```python
from build123d import *

# Parameters (mm, degrees)
F0_W        = 88.9
F0_H        = 165.1
F1_DEPTH    = 6.35
F2_DEPTH    = 25.4
F3_DEPTH    = 50.8
F4_C1_SIZE2 = 7.3323484187
F4_C1_SIZE  = 12.7
F4_C2_SIZE2 = 7.3323484187
F4_C2_SIZE  = 12.7
F4_C3_SIZE2 = 12.7
F4_C3_SIZE  = 7.3323484187
F4_C4_SIZE2 = 12.7
F4_C4_SIZE  = 7.3323484187
F5_R        = 6.34999
F6_C1_SIZE2 = 7.3323484187
F6_C1_SIZE  = 12.7
F6_C2_SIZE2 = 7.3323484187
F6_C2_SIZE  = 12.7
F6_C3_SIZE2 = 12.7
F6_C3_SIZE  = 7.3323484187
F6_C4_SIZE2 = 12.7
F6_C4_SIZE  = 7.3323484187


# Not quite as in the source:
# - a fillet or chamfer is up to 0.001 mm smaller than in the source, because OpenCascade refuses the exact size


with BuildPart() as f1:
    # F0 (on Top) → F1 (new body)
    with BuildSketch(Plane.XY):
        Rectangle(F0_W, F0_H)
        Polygon((0, 76.2), (38.1, 76.2), (38.1, -38.1), (38.1, -76.2), (0, -76.2), (-38.1, -76.2), (-38.1, 38.1), (-38.1, 76.2), align=None, mode=Mode.SUBTRACT)
        with BuildLine():
            Line((0, 50.8), (0, 76.2))
            Line((0, 76.2), (-38.1, 76.2))
            Line((-38.1, 76.2), (-38.1, 38.1))
            Line((-38.1, 38.1), (-12.7, 38.1))
            ThreePointArc((-12.7, 38.1), (-3.7197438789, 41.8197438789), (0, 50.8))
        make_face()
        with BuildLine():
            Line((38.1, -38.1), (38.1, 76.2))
            Line((38.1, 76.2), (0, 76.2))
            Line((0, 76.2), (0, 50.8))
            ThreePointArc((0, 50.8), (-3.7197438789, 41.8197438789), (-12.7, 38.1))
            Line((-12.7, 38.1), (-38.1, 38.1))
            Line((-38.1, 38.1), (-38.1, -76.2))
            Line((-38.1, -76.2), (0, -76.2))
            Line((0, -76.2), (0, -50.8))
            ThreePointArc((0, -50.8), (3.7197438789, -41.8197438789), (12.7, -38.1))
            Line((12.7, -38.1), (38.1, -38.1))
        make_face()
        with BuildLine():
            Line((38.1, -76.2), (38.1, -38.1))
            Line((38.1, -38.1), (12.7, -38.1))
            ThreePointArc((12.7, -38.1), (3.7197438789, -41.8197438789), (0, -50.8))
            Line((0, -50.8), (0, -76.2))
            Line((0, -76.2), (38.1, -76.2))
        make_face()
    extrude(amount=F1_DEPTH)

    # F0 (on Top) → F2 (join)
    with BuildSketch(Plane.XY):
        with BuildLine():
            Line((38.1, -38.1), (38.1, 76.2))
            Line((38.1, 76.2), (0, 76.2))
            Line((0, 76.2), (0, 50.8))
            ThreePointArc((0, 50.8), (-3.7197438789, 41.8197438789), (-12.7, 38.1))
            Line((-12.7, 38.1), (-38.1, 38.1))
            Line((-38.1, 38.1), (-38.1, -76.2))
            Line((-38.1, -76.2), (0, -76.2))
            Line((0, -76.2), (0, -50.8))
            ThreePointArc((0, -50.8), (3.7197438789, -41.8197438789), (12.7, -38.1))
            Line((12.7, -38.1), (38.1, -38.1))
        make_face()
        with BuildLine():
            Line((0, 50.8), (0, 76.2))
            Line((0, 76.2), (-38.1, 76.2))
            Line((-38.1, 76.2), (-38.1, 38.1))
            Line((-38.1, 38.1), (-12.7, 38.1))
            ThreePointArc((-12.7, 38.1), (-3.7197438789, 41.8197438789), (0, 50.8))
        make_face()
        with BuildLine():
            Line((38.1, -76.2), (38.1, -38.1))
            Line((38.1, -38.1), (12.7, -38.1))
            ThreePointArc((12.7, -38.1), (3.7197438789, -41.8197438789), (0, -50.8))
            Line((0, -50.8), (0, -76.2))
            Line((0, -76.2), (38.1, -76.2))
        make_face()
    extrude(amount=F2_DEPTH)

    # F0 (on Top) → F3 (join)
    with BuildSketch(Plane.XY):
        with BuildLine():
            Line((0, 50.8), (0, 76.2))
            Line((0, 76.2), (-38.1, 76.2))
            Line((-38.1, 76.2), (-38.1, 38.1))
            Line((-38.1, 38.1), (-12.7, 38.1))
            ThreePointArc((-12.7, 38.1), (-3.7197438789, 41.8197438789), (0, 50.8))
        make_face()
        with BuildLine():
            Line((38.1, -76.2), (38.1, -38.1))
            Line((38.1, -38.1), (12.7, -38.1))
            ThreePointArc((12.7, -38.1), (3.7197438789, -41.8197438789), (0, -50.8))
            Line((0, -50.8), (0, -76.2))
            Line((0, -76.2), (38.1, -76.2))
        make_face()
    extrude(amount=F3_DEPTH)

    # F4: chamfer of 12.7 x 7.3323484187 on 4 edges, made by hand

    # F4_c1
    f4_c1_edges = [f1.edges().sort_by_distance(p)[0] for p in [
        (-19.05, -76.2, 25.4),
    ]]
    f4_c1_side = f1.faces().sort_by_distance((-19.05, -76.2, 25.2533530316))[0]
    chamfer(f4_c1_edges, length=F4_C1_SIZE, length2=F4_C1_SIZE2, reference=f4_c1_side)

    # F4_c2
    f4_c2_edges = [f1.edges().sort_by_distance(p)[0] for p in [
        (38.1, 19.05, 25.4),
    ]]
    f4_c2_side = f1.faces().sort_by_distance((38.1, 19.05, 25.2533530316))[0]
    chamfer(f4_c2_edges, length=F4_C2_SIZE, length2=F4_C2_SIZE2, reference=f4_c2_side)

    # F4_c3
    f4_c3_edges = [f1.edges().sort_by_distance(p)[0] for p in [
        (-38.1, -15.3838257906, 25.4),
    ]]
    f4_c3_side = f1.faces().sort_by_distance((-37.9533530316, -15.3838257906, 25.4))[0]
    chamfer(f4_c3_edges, length=F4_C3_SIZE, length2=F4_C3_SIZE2, reference=f4_c3_side)

    # F4_c4
    f4_c4_edges = [f1.edges().sort_by_distance(p)[0] for p in [
        (15.3838257906, 76.2, 25.4),
    ]]
    f4_c4_side = f1.faces().sort_by_distance((15.3838257906, 76.0533530316, 25.4))[0]
    chamfer(f4_c4_edges, length=F4_C4_SIZE, length2=F4_C4_SIZE2, reference=f4_c4_side)

    # F5 (radius 6.35 in the source; OpenCascade refuses exactly that, so slightly less here)
    f5_edges = [f1.edges().sort_by_distance(p)[0] for p in [
        (0, 82.55, 6.35),
        (44.45, 0, 6.35),
        (-44.45, 0, 6.35),
        (0, -82.55, 6.35),
    ]]
    fillet(f5_edges, radius=F5_R)

    # F6: chamfer of 12.7 x 7.3323484187 on 4 edges, made by hand

    # F6_c1
    f6_c1_edges = [f1.edges().sort_by_distance(p)[0] for p in [
        (-38.1, 57.15, 50.8),
    ]]
    f6_c1_side = f1.faces().sort_by_distance((-38.1, 57.15, 50.6533530316))[0]
    chamfer(f6_c1_edges, length=F6_C1_SIZE, length2=F6_C1_SIZE2, reference=f6_c1_side)

    # F6_c2
    f6_c2_edges = [f1.edges().sort_by_distance(p)[0] for p in [
        (-15.3838257906, 76.2, 50.8),
    ]]
    f6_c2_side = f1.faces().sort_by_distance((-15.3838257906, 76.2, 50.6533530316))[0]
    chamfer(f6_c2_edges, length=F6_C2_SIZE, length2=F6_C2_SIZE2, reference=f6_c2_side)

    # F6_c3
    f6_c3_edges = [f1.edges().sort_by_distance(p)[0] for p in [
        (38.1, -57.15, 50.8),
    ]]
    f6_c3_side = f1.faces().sort_by_distance((38.1, -57.15, 50.6533530316))[0]
    chamfer(f6_c3_edges, length=F6_C3_SIZE, length2=F6_C3_SIZE2, reference=f6_c3_side)

    # F6_c4
    f6_c4_edges = [f1.edges().sort_by_distance(p)[0] for p in [
        (12.7, -76.2, 50.8),
    ]]
    f6_c4_side = f1.faces().sort_by_distance((12.7, -76.2, 50.6533530316))[0]
    chamfer(f6_c4_edges, length=F6_C4_SIZE, length2=F6_C4_SIZE2, reference=f6_c4_side)


solid = f1.part
```
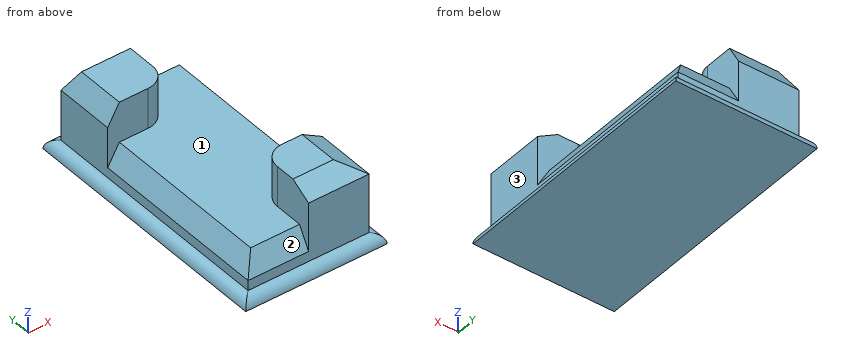
For this review, take the finished solid that the model builds, in its own axes (mm). Face numbers are marked on the shaded views. A direction names the side the tool comes from. Give positions to 0.01 mm unless a question says otherwise; leave off trailing zeros. Order: outer loops, then holes, each group sorted by start corner. A loop starts at its lowest first (then second) coordinate and runs counter-clockwise, first axis right, second up.
1) Insertion check: pin 1 (5 mm diameter, centred on y = -42, z = 32.5, fed in from +X); pin 2 (7.5 mm diameter, centred on x = 20.5, z = 29, fed in from +Y); pin 3 (4 mm diameter, centred on x = -10.5, z = 11.5, fed in from +Y). Each pin has a flat end and moves straight along its axis. Give the tip position at first contact, or say it passes through.
2) Take a section at A-A (z = 32). Give the boundary of the cut face in (x, y), then the cut area to 3 significant figures.
3) Take a section at D-D (z = 16.5). Give the boundary of the cut face in (x, y).
4) Wall thickness on line 1 (Y direction, x = 16, z = 7.5); line 2 (Z direction, x = -19, y = 22.5); line 3 (X direction, y = -53.5, z = 37): over which ranges is each line inside the solid? List them lowest first.
5) For the marked faces 1, 2 and 3, list the 3-axis set-ups (+Z, -Z, +X, -X, +Y, -Y) from which the entire face can be reached by the end or side of a thin tool; tool diameter is ignored.
Derived:
1. pin 1: stops at x = 38.1
1. pin 2: stops at y = 68.95
1. pin 3: stops at y = 76.2
2. outline: (-38.1, 38.1) - (-12.7, 38.1) arc R12.7 ccw to (0, 50.8) - (0, 76.2) - (-38.1, 76.2) - close; (0, -76.2) - (38.1, -76.2) - (38.1, -38.1) - (12.7, -38.1) arc R12.7 ccw to (0, -50.8) - close
2. area: 2,830 mm2
3. outline: (-38.1, 38.1) - (-35.91, 38.1) - (-35.91, -74.01) - (0, -74.01) - (0, -76.2) - (38.1, -76.2) - (38.1, -38.1) - (35.91, -38.1) - (35.91, 74.01) - (0, 74.01) - (0, 76.2) - (-38.1, 76.2) - close
4. line 1: y = -76.2 to 76.2
4. line 2: z = 0 to 25.4
4. line 3: x = 0 to 38.1
5. face 1: +Z
5. face 2: +Z, -X, -Y
5. face 3: +Z, +X, +Y, -Y
